Check sheet for the modelled part. Datum: model origin and axes. Units: mm. Round coordinates to 2 decimals unless told otherwise and drop trailing zeros. Order: outer loops, then holes, each group sorted by start corner. A loop starts at its lowest first (then second) coordinate and runs counter-clockwise, first axis right, second up. Notation, with made-up numbers: (83, 63) -> (98, 63) arc R22 cw to (98, 92) -> close; hole circle Ø3 at (66.5, 76.25). An arc over 180 degrees is marked (long way). Answer in a Markdown table with one row per item.
from build123d import *

# Parameters (mm, degrees)
SKETCH1_W                        = 25.4
SKETCH1_H                        = 25.4
SKETCH1_W_2                      = 22.225
SKETCH1_H_2                      = 22.225
BOSS_EXTRUDE1_DEPTH              = 254
F_10_0_1935_DIAMETER_HOLE1_D     = 4.9149
F_10_0_1935_DIAMETER_HOLE1_DEPTH = 50.8
F_10_0_1935_DIAMETER_HOLE1_TIP   = 1.476584928
SKETCH5_R                        = 1.778
CUT_EXTRUDE1_DEPTH               = 256.582569828


with BuildPart() as part:
    # Sketch1 → Boss-Extrude1 (new, symmetric)
    with BuildSketch(Plane(origin=(0, 0, 0), x_dir=(1, 0, 0), z_dir=(0, 1, 0))):
        Rectangle(SKETCH1_W, SKETCH1_H)
        Rectangle(SKETCH1_W_2, SKETCH1_H_2, mode=Mode.SUBTRACT)
    extrude(amount=BOSS_EXTRUDE1_DEPTH, both=True)

    # #10 (0.1935) Diameter Hole1
    with Locations(Plane(origin=(0, 0, -12.7), x_dir=(-1, 0, 0), z_dir=(0, 0, -1))):
        with Locations((0, 228.6), (0, -228.6)):
            Hole(F_10_0_1935_DIAMETER_HOLE1_D / 2, depth=F_10_0_1935_DIAMETER_HOLE1_DEPTH)
            with Locations((0, 0, -(F_10_0_1935_DIAMETER_HOLE1_DEPTH + F_10_0_1935_DIAMETER_HOLE1_TIP / 2))):  # 118° drill point
                Cone(0, F_10_0_1935_DIAMETER_HOLE1_D / 2, F_10_0_1935_DIAMETER_HOLE1_TIP, mode=Mode.SUBTRACT)

    # Sketch5 → Cut-Extrude1 (cut, through all)
    with BuildSketch(Plane.XY.offset(12.7)):
        with Locations((0, 190.5)):
            Circle(SKETCH5_R)
        with Locations((0, 139.7)):
            Circle(SKETCH5_R)
        with Locations((0, 177.8)):
            Circle(SKETCH5_R)
        with Locations((0, 165.1)):
            Circle(SKETCH5_R)
        with Locations((0, 152.4)):
            Circle(SKETCH5_R)
        with Locations((0, 127)):
            Circle(SKETCH5_R)
        with Locations((0, 114.3)):
            Circle(SKETCH5_R)
    cut_extrude1 = extrude(amount=-CUT_EXTRUDE1_DEPTH, mode=Mode.SUBTRACT)

    # Mirror1: Cut-Extrude1 across plane
    add(cut_extrude1.mirror(Plane.ZX), mode=Mode.SUBTRACT)


solid = part.part
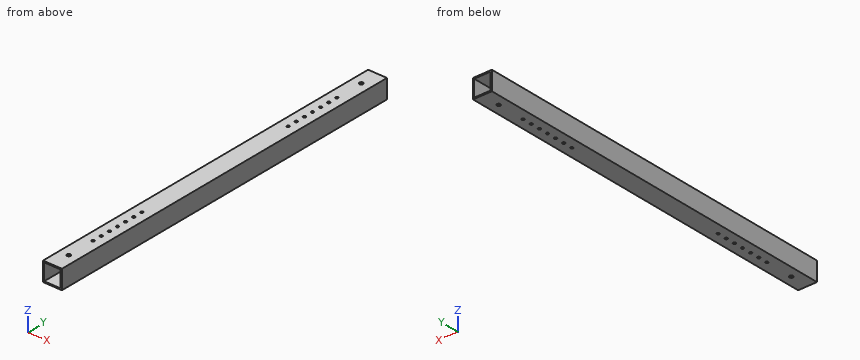
Item 1: Scan lines: line 1 (X direction, y = 150, z = 6.75); line 2 (X direction, y = -228.6, z = 11.9). Record each from-to range of solid material in increasing order. Write a range as [from, to].
Result sheet:
| item | result |
|---|---|
| line 1 | x = [-12.7, -11.11], [11.11, 12.7] |
| line 2 | x = [-12.7, -2.46], [2.46, 12.7] |
Item 2: Cross-section at A-A (y = 212). Record the boundary of the cut face in (x, z), and give its area (3 significant figures).
Result sheet:
| item | result |
|---|---|
| outline | (-12.7, -12.7) -> (12.7, -12.7) -> (12.7, 12.7) -> (-12.7, 12.7) -> close; hole (-11.11, -11.11) -> (11.11, -11.11) -> (11.11, 11.11) -> (-11.11, 11.11) -> close |
| area | 151 mm^2 |
Item 3: Cross-section at B-B (z = 4). Record the boundary of the cut face in (x, y), and give its area (3 significant figures).
Result sheet:
| item | result |
|---|---|
| outline | (-12.7, -254) -> (-11.11, -254) -> (-11.11, 254) -> (-12.7, 254) -> close; (11.11, -254) -> (12.7, -254) -> (12.7, 254) -> (11.11, 254) -> close |
| area | 1,610 mm^2 |
